The drawing under review shows one solid part. Ordinate dimensions are in mm from its lowest x, y, z. A direction names the side the tool comes from. Coordinates: 2 decimals unless noted, no trailing zeros. Loops run counter-clockwise (first coordinate to the right, second up) from the corner with the lowest first, then second, coordinate; pieces in that order, holes last. Notation, with made-up numbers: (55.5, -28.5) -> (85.5, -28.5) arc R7 cw to (85.5, -19.5) -> close; hole circle Ø11 at (-31, 58). An arc over 180 degrees is marked (long way). Use a Markdown table: item, result.
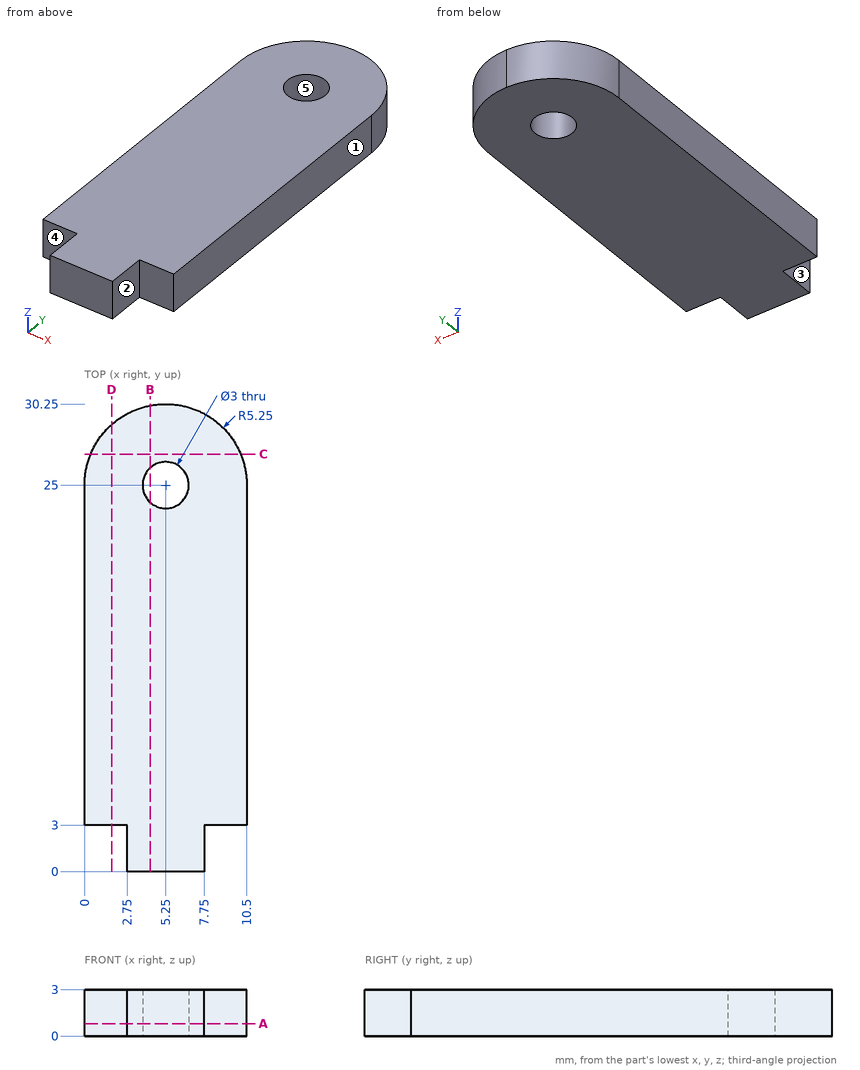
(1) For line 1 along X through (y, z) = (25, 0.8); line 2 along Y through (x, z) = (4.5, 2.8); line 3 along Y through (x, z) = (7.5, 0.5), list the stretches that pass through material, from the lowest coordinate up.
Found:
| item | result |
|---|---|
| line 1 | x = 0 to 3.75, 6.75 to 10.5 |
| line 2 | y = 0 to 23.7, 26.3 to 30.2 |
| line 3 | y = 0 to 29.74 |
(2) Mouldability with a two-part tool opening along X and no side actions: class the marked faces 3, 4 and 5 as pulls with the +X half, pulls with the -X half, needs draft (parallel to the pull), parting line crosses it, or undercut.
Found:
| item | result |
|---|---|
| face 3 | pulls with the -X half |
| face 4 | needs draft |
| face 5 | undercut |
(3) For the marked faces 1 and 2, list the 3-axis set-ups (+Z, -Z, +X, -X, +Y, -Y) from which the entire face can be reached by the end or side of a thin tool; tool diameter is ignored.
Found:
| item | result |
|---|---|
| face 1 | +Z, -Z, +X, +Y, -Y |
| face 2 | +Z, -Z, +X, -Y |
(4) For pin 1 Ø4 at (x, y) = (5.25, 25) entering from -Z; pin 2 Ø1.4 at (x, z) = (8.5, 2) entering from -Y; pin 3 Ø0.9 at (y, z) = (1.5, 2) entering from -X; pin 4 Ø0.9 at (y, z) = (2, 2) entering from +X, all flat-tipped, find the tip position at first contact; note any pin that passes through.
Found:
| item | result |
|---|---|
| pin 1 | stops at z = 0 |
| pin 2 | stops at y = 3 |
| pin 3 | stops at x = 2.75 |
| pin 4 | stops at x = 7.75 |
(5) Take a section at D-D on x = 1.75. Write out the cut boundary in (y, z).
Found:
| item | result |
|---|---|
| outline | (3, 0) -> (28.91, 0) -> (28.91, 3) -> (3, 3) -> close |
(6) Take a section at A-A on z = 0.8. Write out the cut boundary in (x, y).
Found:
| item | result |
|---|---|
| outline | (0, 3) -> (2.75, 3) -> (2.75, 0) -> (7.75, 0) -> (7.75, 3) -> (10.5, 3) -> (10.5, 25) arc R5.25 ccw to (0, 25) -> close; hole circle Ø3 at (5.25, 25) |
(7) Take a section at B-B on x = 4.25. Write out the cut boundary in (y, z), plus the area to 3 significant figures.
Found:
| item | result |
|---|---|
| outline | (0, 0) -> (23.88, 0) -> (23.88, 3) -> (0, 3) -> close; (26.12, 0) -> (30.15, 0) -> (30.15, 3) -> (26.12, 3) -> close |
| area | 83.8 mm^2 |
(8) Take a section at C-C on y = 27. Write out the cut boundary in (x, z).
Found:
| item | result |
|---|---|
| outline | (0.4, 0) -> (10.1, 0) -> (10.1, 3) -> (0.4, 3) -> close |
